Can you work these out from the model? Positions are in its coordinate system, mm. A direction names the side the tool comes from. Coordinates: 2 decimals unless noted, no trailing zeros. Write each loop counter-clockwise with the first axis right and the second up, starting at its lowest first coordinate (ties: lowest second). Pieces come first, ordered by that corner, then holes.
```python
from build123d import *

# Parameters (mm, degrees)
MODEL_R                 = 1.25
BOSS_EXTRUDE1_DEPTH     = 2
BOSS_EXTRUDE2_DEPTH     = 11.50072
SKETCH2_R               = 1.25
CUT_EXTRUDE1_DEPTH      = 2
CUT_EXTRUDE1_DEPTH_BACK = 4
SKETCH3_W               = 9.00072
SKETCH3_H               = 2
SKETCH3_W_2             = 8.40072
SKETCH3_H_2             = 1.4
CUT_EXTRUDE2_DEPTH      = 4


with BuildPart() as part:
    # Model → Boss-Extrude1 (new body)
    with BuildSketch(Plane.XY):
        Polygon((1.25, 4), (0, 4), (0, 8), (1.25, 8), (1.25, 12), (10.25072, 12), (10.25072, 8), (11.50072, 8), (11.50072, 4), (10.25072, 4), (10.25072, 0), (1.25, 0), align=None)
        with Locations((7.75072, 6)):
            Circle(MODEL_R, mode=Mode.SUBTRACT)
        with Locations((3.75, 6)):
            Circle(MODEL_R, mode=Mode.SUBTRACT)
    extrude(amount=BOSS_EXTRUDE1_DEPTH)

    # Sketch1 → Boss-Extrude2 (add)
    with BuildSketch(Plane.ZY):
        with BuildLine():
            Line((2, 4), (2, 5))
            ThreePointArc((2, 5), (2.292893219, 4.292893219), (3, 4))
            Line((3, 4), (2, 4))
        make_face()
        with BuildLine():
            Line((0, 4), (-1, 4))
            ThreePointArc((-1, 4), (-0.292893219, 4.292893219), (0, 5))
            Line((0, 5), (0, 4))
        make_face()
    extrude(amount=-BOSS_EXTRUDE2_DEPTH)

    # Sketch2 → Cut-Extrude1 (cut, two sides)
    with BuildSketch(Plane.XY.offset(2)) as cut_extrude1_sk:
        with Locations((3.75, 6)):
            Circle(SKETCH2_R)
        with Locations((7.75072, 6)):
            Circle(SKETCH2_R)
    extrude(amount=CUT_EXTRUDE1_DEPTH, mode=Mode.SUBTRACT)
    extrude(cut_extrude1_sk.sketch, amount=-CUT_EXTRUDE1_DEPTH_BACK, mode=Mode.SUBTRACT)

    # Sketch3 → Cut-Extrude2 (cut)
    with BuildSketch(Plane(origin=(0, 12, 0), x_dir=(1, 0, 0), z_dir=(0, 1, 0))):
        with Locations((5.75036, -1)):
            Rectangle(SKETCH3_W, SKETCH3_H)
        with Locations((5.75036, -1)):
            Rectangle(SKETCH3_W_2, SKETCH3_H_2, mode=Mode.SUBTRACT)
    extrude(amount=-CUT_EXTRUDE2_DEPTH, mode=Mode.SUBTRACT)


solid = part.part
```
1. Which directions (+Z, -Z, +X, -X, +Y, -Y) give clear straight access to the entire face, cutting with the end or side of a thin tool? Please do faces 4 (the face through (6, 7, 0)), 5 (the face through (1.55, 10, 1)), 6 (the face through (6, 10, 1.7)).
2. If we section it at C-C, the plane x = 9.5: List the corners of the cut face in (y, z) for me, plus the area to 3 significant figures.
3. If we section it at D-D, the plane z = 2.4: List the corners of the cut face in (x, y) for me, plus the area to 3 significant figures.
4. If I drill on L1, parallel to X at y = 6, z = 1.05; L2, parallel to Z at x = 8, y = 1.75; L3, parallel to Y at x = 0.5, z = 1.9, over which ranges is the centre line in solid material (lowest first)?
5. I'm going to push flat-ended pins straight in: P1, Ø4.5, axis at x = 7, y = 1, coming from the -Z side; P2, Ø4, axis at x = 4.5, y = 10.5, coming from the +Z side; P3, Ø3, axis at x = 7.75, y = 6, coming from the +Z side. Where does each tip first touch, or does it pass through?
6. We'd pull the mould along X, two halves only. Please class faces 1 (the face through (1.25, 2, 1)), 2 (the face through (7, 5, 1)), 3 (the face through (6, 10, 0.3)): released by +X, released by -X, zero draft, split by the parting line, or undercut.
7. If we section it at B-B, the plane y = 6: List the corners of the cut face in (x, z) for me.
8. If we section it at A-A, the plane x = 3.75: List the corners of the cut face in (y, z) for me.
Answers:
1. face 4: -Z, +X, -X, +Y
1. face 5: +Z, -Z, -X, +Y
1. face 6: +Z, +X, -X, +Y
2. outline: (0, 0) - (4, 0) - (4, -1) arc R1 cw to (5, 0) - (8, 0) - (8, 0.3) - (12, 0.3) - (12, 1.7) - (8, 1.7) - (8, 2) - (5, 2) arc R1 cw to (4, 3) - (4, 2) - (0, 2) - close
2. area: 22.0 mm2
3. outline: (0, 4) - (11.5, 4) - (11.5, 4.2) - (0, 4.2) - close
3. area: 2.30 mm2
4. L1: x = 0 to 2.5, 5 to 6.5, 9 to 11.5
4. L2: z = 0 to 2
4. L3: y = 4 to 8
5. P1: stops at z = 0
5. P2: stops at z = 1.7
5. P3: stops at z = 2.13
6. face 1: released by -X
6. face 2: undercut
6. face 3: zero draft
7. outline: (0, 0) - (2.5, 0) - (2.5, 2) - (0, 2) - close; (5, 0) - (6.5, 0) - (6.5, 2) - (5, 2) - close; (9, 0) - (11.5, 0) - (11.5, 2) - (9, 2) - close
8. outline: (0, 0) - (4, 0) - (4, -1) arc R1 cw to (4.75, -0.03) - (4.75, 2.03) arc R1 cw to (4, 3) - (4, 2) - (0, 2) - close; (7.25, 0) - (8, 0) - (8, 0.3) - (12, 0.3) - (12, 1.7) - (8, 1.7) - (8, 2) - (7.25, 2) - close
